Geometry: see drawing. Coordinates: mm, zero at the bounding-box minimum. Round coordinates to 2 decimals unless told otherwise and drop trailing zeros. Loops run counter-clockwise (first coordinate to the right, second up) from the corner with the lowest first, then second, coordinate; pieces in that order, holes last.
(1) Mould query, pull axis Z, two halves, no side actions, for the marked faces 1, 2 and 3. Classes: pulls with the +Z half, pulls with the -Z half, needs draft (parallel to the pull), parting line crosses it, or undercut.
(2) Section D-D, the plane z = 9. Return the cut outline in (x, y).
(3) First-contact query: pin 1 Ø2.5 at (x, z) = (9.37, 26.9) entering from +Y; pin 2 Ø3 at (x, y) = (22, 10.5) entering from -Z; pin 3 Ø8 at (x, z) = (17, 17) entering from -Y; pin 4 Ø1 at (y, z) = (5, 13) entering from +X. Flat tips, straight axial feed; report the tip coordinate or a pass-through.
(4) Section B-B, the plane y = 3.75. Return the cut outline in (x, z), plus the area to 3 significant figures.
(5) Section A-A, the plane x = 17. Return the cut outline in (y, z).
(6) Section C-C, the plane z = 4.5. Return the cut outline in (x, y) (1 decimal), plus the area to 3 significant figures.
(7) Material intervals for probe 1 along X at (y, z) = (3, 14.5) (1 decimal); probe 2 along X at (y, z) = (3.75, 18.5) (1 decimal); probe 3 along X at (y, z) = (5.5, 17), sorted ascending.
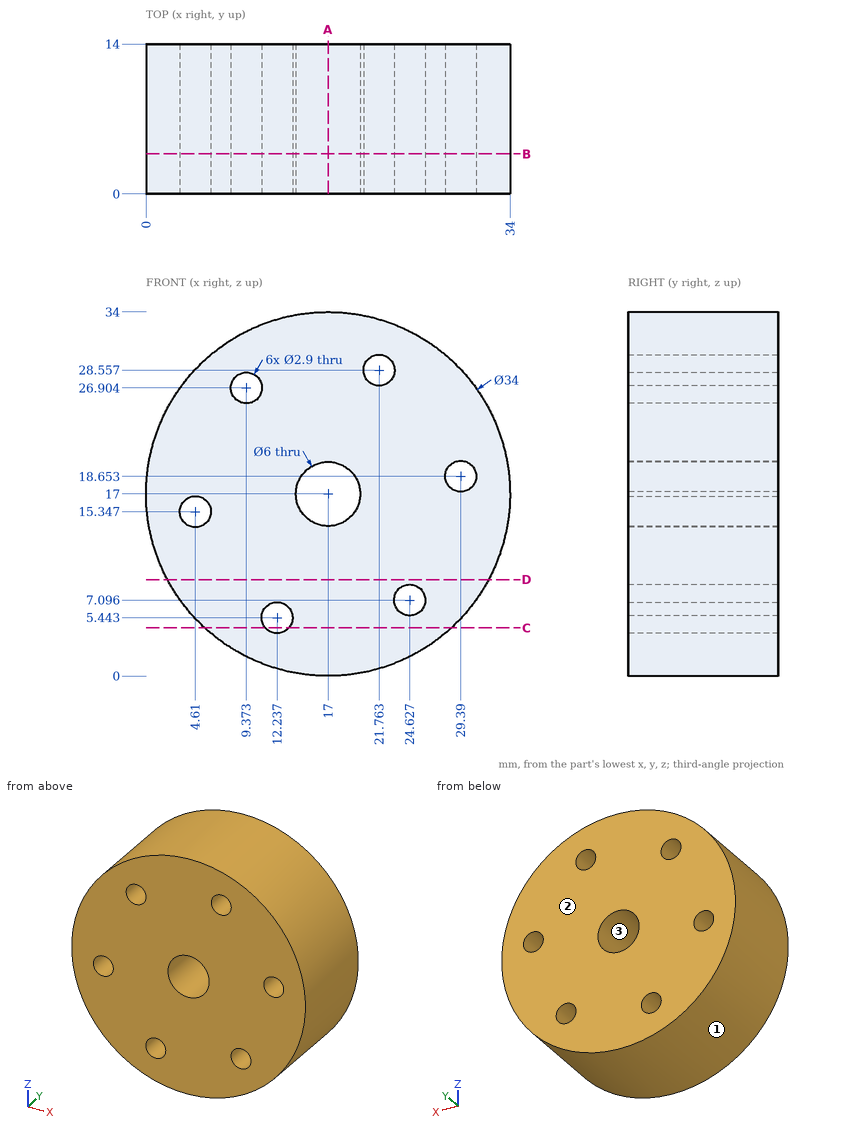
Output values:
1. face 1: parting line crosses it
1. face 2: needs draft
1. face 3: undercut
2. outline: (2, 0) - (32, 0) - (32, 14) - (2, 14) - close
3. pin 1: passes through
3. pin 2: stops at z = 0.36
3. pin 3: stops at y = 0
3. pin 4: stops at x = 33.64
4. outline: circle Ø34 at (17, 17); hole circle Ø2.9 at (4.61, 15.35); hole circle Ø2.9 at (9.37, 26.9); hole circle Ø2.9 at (12.24, 5.44); hole circle Ø6 at (17, 17); hole circle Ø2.9 at (21.76, 28.56); hole circle Ø2.9 at (24.63, 7.1); hole circle Ø2.9 at (29.39, 18.65)
4. area: 840 mm2
5. outline: (0, 0) - (14, 0) - (14, 14) - (0, 14) - close; (0, 20) - (14, 20) - (14, 34) - (0, 34) - close
6. outline: (5.5, 0) - (11.1, 0) - (11.1, 14) - (5.5, 14) - close; (13.3, 0) - (28.5, 0) - (28.5, 14) - (13.3, 14) - close
6. area: 292 mm2
7. probe 1: x = 0.2 to 3.4, 5.8 to 15.3, 18.7 to 33.8
7. probe 2: x = 0.1 to 14.4, 19.6 to 27.9, 30.8 to 33.9
7. probe 3: x = 0 to 14, 20 to 34
